Part model, mm, in its own coordinate system. A direction names the side the tool comes from. Round coordinates to 2 decimals unless told otherwise and drop trailing zeros. Write each loop counter-clockwise with the first axis right and the second up, starting at its lowest first coordinate (ties: lowest second). Pieces come first, ordered by that corner, then holes.
1) Which spindle directions (+Z, -Z, +X, -X, +Y, -Y) get a long thin tool onto all of the face, cutting with end or side? Do faces 4 (the flat face through (-8.5, 88, 0)), 5 (the flat face through (-3, 88, -10)), 6 (the flat face through (-9, 5, 2)). Say none if no direction does.
2) Drill centre lines: L1, parallel to X at y = 152, z = 0; L2, parallel to X at y = 2.05, z = 0; L3, parallel to X at y = 102, z = -2. Where is each one in solid material? Low to high.
3) Flat gauge pins, fed straight in: pin 1 (2.5 mm diameter, centred on x = -9.5, y = 61.5, fed in from +Z); pin 2 (4 mm diameter, centred on y = 62, z = -3.5, fed in from -X); pin 3 (1.7 mm diameter, centred on y = 110.5, z = -10.5, fed in from -X). Where does each tip first touch, or does it go through?
4) Saw through at C-C on z = 22. Write the cut outline in (x, y).
5) Saw through at A-A on y = 146.5. Write the cut outline in (x, z), and give its area (3 significant figures).
6) Pull direction Z, two halves, no side cores. Call faces 1 (the cylindrical face through (-19, 1.5, 12.4)), 2 (the flat face through (11, 9, -7)), 3 (the flat face through (0, 88, 8.5)): +Z half, -Z half, draft (parallel to the pull), parting line (faces both ways), or undercut.
7) Saw through at D-D on y = 90. Write the cut outline in (x, z), and give its area (3 significant figures).
```python
from build123d import *

# Parameters (mm, degrees)
ESBO_O1_R                = 28
RESSALTO_EXTRUS_O1_DEPTH = 5
ESBO_O6_R                = 10.75
CORTE_EXTRUS_O1_DEPTH    = 5
ESBO_O7_R                = 9
CORTE_EXTRUS_O2_DEPTH    = 0.4
CORTE_EXTRUS_O3_REACH    = 161.978
ESBO_O8_R                = 3.05
PADR_OCIRCULAR1_COUNT    = 3
CORTE_EXTRUS_O4_REACH    = 161.978
ESBO_O9_R                = 1.4
PADR_OCIRCULAR2_COUNT    = 3
PADR_OCIRCULAR3_COUNT    = 3
CHANFRO1_SIZE            = 2
CHANFRO2_SIZE            = 2
CORTE_EXTRUS_O5_DEPTH    = 136
PADR_OCIRCULAR4_COUNT    = 4
ESBO_O18_R               = 2.5
CORTE_EXTRUS_O6_DEPTH    = 10


with BuildPart() as part:
    # Esboço1 → Ressalto-extrusão1 (new body)
    with BuildSketch(Plane(origin=(0, 0, 0), x_dir=(1, 0, 0), z_dir=(0, 1, 0))):
        with Locations(Location((0, 0, 0), (0, 0, 270))):
            Circle(ESBO_O1_R)
    extrude(amount=RESSALTO_EXTRUS_O1_DEPTH)

    # Esboço5 → Revolução1 (revolve)
    with BuildSketch(Plane(origin=(0, 0, 0), x_dir=(0, 0, -1), z_dir=(1, 0, 0))):
        Polygon((0, 5), (-16.5, 5), (-14.5, 7), (-14.5, 9), (-12.3, 9), (-12.3, 155), (0, 155), align=None)
    revolve(axis=Axis((0, 155, 0), (0, -1, 0)))

    # Esboço6 → Corte-extrusão1 (cut)
    with BuildSketch(Plane.XZ):
        with Locations(Location((0, 0, 0), (0, 0, 270))):
            Circle(ESBO_O6_R)
    extrude(amount=-CORTE_EXTRUS_O1_DEPTH, mode=Mode.SUBTRACT)

    # Esboço7 → Corte-extrusão2 (cut)
    with BuildSketch(Plane.XZ.offset(-5)):
        with Locations(Location((0, 0, 0), (0, 0, 270))):
            Circle(ESBO_O7_R)
    extrude(amount=-CORTE_EXTRUS_O2_DEPTH, mode=Mode.SUBTRACT)

    # Esboço8 → Corte-extrusão3 (cut, up to next)
    with BuildSketch(Plane.XZ, mode=Mode.PRIVATE) as corte_extrus_o3_sk1:
        with Locations(Location((0, 22.5, 0), (0, 0, 270))):
            Circle(ESBO_O8_R)
    corte_extrus_o3_tool1 = extrude(corte_extrus_o3_sk1.sketch, amount=-CORTE_EXTRUS_O3_REACH, mode=Mode.PRIVATE) & part.part
    corte_extrus_o3 = corte_extrus_o3_tool1.solids().sort_by_distance((0, 0, 22.5))[0]
    add(corte_extrus_o3, mode=Mode.SUBTRACT)

    # PadrãoCircular1: Corte-extrusão3 ×3 about axis
    padr_ocircular1_axis = Axis((0, 0, 0), (0, 1, 0))
    for i in range(1, PADR_OCIRCULAR1_COUNT):
        add(corte_extrus_o3.rotate(padr_ocircular1_axis, i * 360 / PADR_OCIRCULAR1_COUNT), mode=Mode.SUBTRACT)

    # Esboço9 → Corte-extrusão4 (cut, up to next)
    with BuildSketch(Plane.XZ, mode=Mode.PRIVATE) as corte_extrus_o4_sk1:
        with Locations(Location((-19.052558883, 11, 0), (0, 0, 270))):
            Circle(ESBO_O9_R)
    corte_extrus_o4_tool1 = extrude(corte_extrus_o4_sk1.sketch, amount=-CORTE_EXTRUS_O4_REACH, mode=Mode.PRIVATE) & part.part
    corte_extrus_o4 = corte_extrus_o4_tool1.solids().sort_by_distance((-19.052559, 0, 11))[0]
    add(corte_extrus_o4, mode=Mode.SUBTRACT)

    # PadrãoCircular2: Corte-extrusão4 ×3 about axis
    padr_ocircular2_axis = Axis((0, 0, 0), (0, 1, 0))
    for i in range(1, PADR_OCIRCULAR2_COUNT):
        add(corte_extrus_o4.rotate(padr_ocircular2_axis, i * 360 / PADR_OCIRCULAR2_COUNT), mode=Mode.SUBTRACT)

    # Loft de corte1: read off the stored shape, not the designer's step
    # Loft de corte1: loft between two sections, ruled curve by curve
    loft_de_corte1_from = [
        Edge.make_bspline([(-18.260331243, 3, 17.20543513), (-17.315862444, 3, 16.040111704), (-16.150539018, 3, 16.984580503), (-17.095007817, 3, 18.149903929), (-18.039476615, 3, 19.315227355), (-19.204800042, 3, 18.370758556), (-18.260331243, 3, 17.20543513)], [0, 0, 0, 0, 0.5, 0.5, 0.5, 1, 1, 1, 1], 3, [1, 0.333333333, 0.333333333, 1, 0.333333333, 0.333333333, 1]),
    ]
    loft_de_corte1_to = [
        Edge.make_bspline([(-18.914864913, 0, 17.499210616), (-18.557947085, 0, 15.024819849), (-16.083556319, 0, 15.381737677), (-16.440474147, 0, 17.856128444), (-16.797391974, 0, 20.33051921), (-19.271782741, 0, 19.973601382), (-18.914864913, 0, 17.499210616)], [0, 0, 0, 0, 0.5, 0.5, 0.5, 1, 1, 1, 1], 3, [1, 0.333333333, 0.333333333, 1, 0.333333333, 0.333333333, 1]),
    ]
    loft_de_corte1 = Solid(Shell([*[Face.make_surface_from_curves(loft_de_corte1_from[k], loft_de_corte1_to[k]) for k in range(1)], Face(Wire(loft_de_corte1_from)), Face(Wire(loft_de_corte1_to))]))
    add(loft_de_corte1, mode=Mode.SUBTRACT)

    # PadrãoCircular3: Loft de corte1 ×3 about axis
    padr_ocircular3_axis = Axis((0, 0, 0), (0, 1, 0))
    for i in range(1, PADR_OCIRCULAR3_COUNT):
        add(loft_de_corte1.rotate(padr_ocircular3_axis, i * 360 / PADR_OCIRCULAR3_COUNT), mode=Mode.SUBTRACT)

    # Chanfro1
    chanfro1_edges = [part.edges().sort_by_distance(p)[0] for p in [
        (-19.052558883, 5, 12.4),
    ]]
    chamfer(chanfro1_edges, length=CHANFRO1_SIZE)

    # Chanfro2
    chanfro2_edges = [part.edges().sort_by_distance(p)[0] for p in [
        (20.264994449, 5, 10.3),
        (-1.212435565, 5, -22.7),
    ]]
    chamfer(chanfro2_edges, length=CHANFRO2_SIZE)

    # Esboço17 → Corte-extrusão5 (cut)
    with BuildSketch(Plane(origin=(0, 155, 0), x_dir=(1, 0, 0), z_dir=(0, 1, 0))):
        with BuildLine():
            Line((-3, 8.5), (3, 8.5))
            Line((3, 8.5), (3, 11.928537211))
            ThreePointArc((3, 11.928537211), (0, 12.3), (-3, 11.928537211))
            Line((-3, 11.928537211), (-3, 8.5))
        make_face()
    corte_extrus_o5 = extrude(amount=-CORTE_EXTRUS_O5_DEPTH, mode=Mode.SUBTRACT)

    # PadrãoCircular4: Corte-extrusão5 ×4 about axis
    padr_ocircular4_axis = Axis((0, 0, 0), (0, 1, 0))
    for i in range(1, PADR_OCIRCULAR4_COUNT):
        add(corte_extrus_o5.rotate(padr_ocircular4_axis, i * 360 / PADR_OCIRCULAR4_COUNT), mode=Mode.SUBTRACT)

    # Esboço18 → Corte-extrusão6 (cut)
    with BuildSketch(Plane(origin=(0, 155, 0), x_dir=(1, 0, 0), z_dir=(0, 1, 0))):
        with Locations(Location((0, 0, 0), (0, 0, 270))):
            Circle(ESBO_O18_R)
    extrude(amount=-CORTE_EXTRUS_O6_DEPTH, mode=Mode.SUBTRACT)


solid = part.part
```
Completed:
1. face 4: -X, +Y
1. face 5: -Z, +Y
1. face 6: -Y
2. L1: x = -8.5 to -2.5, 2.5 to 8.5
2. L2: x = -28 to -10.75, 10.75 to 28
2. L3: x = -8.5 to 8.5
3. pin 1: stops at z = 9.12
3. pin 2: stops at x = -11.93
3. pin 3: stops at x = -7.63
4. outline: (-17.32, 0) - (-3.01, 0) - (-3.01, 5) - (-17.32, 5) - close; (3.01, 0) - (17.32, 0) - (17.32, 5) - (3.01, 5) - close
5. outline: (-11.93, -3) arc R12.3 ccw to (-3, -11.93) - (-3, -8.5) - (3, -8.5) - (3, -11.93) arc R12.3 ccw to (11.93, -3) - (8.5, -3) - (8.5, 3) - (11.93, 3) arc R12.3 ccw to (3, 11.93) - (3, 8.5) - (-3, 8.5) - (-3, 11.93) arc R12.3 ccw to (-11.93, 3) - (-8.5, 3) - (-8.5, -3) - close; hole circle Ø5 at (0, 0)
5. area: 367 mm2
6. face 1: undercut
6. face 2: draft
6. face 3: +Z half
7. outline: (-11.93, -3) arc R12.3 ccw to (-3, -11.93) - (-3, -8.5) - (3, -8.5) - (3, -11.93) arc R12.3 ccw to (11.93, -3) - (8.5, -3) - (8.5, 3) - (11.93, 3) arc R12.3 ccw to (3, 11.93) - (3, 8.5) - (-3, 8.5) - (-3, 11.93) arc R12.3 ccw to (-11.93, 3) - (-8.5, 3) - (-8.5, -3) - close
7. area: 387 mm2
